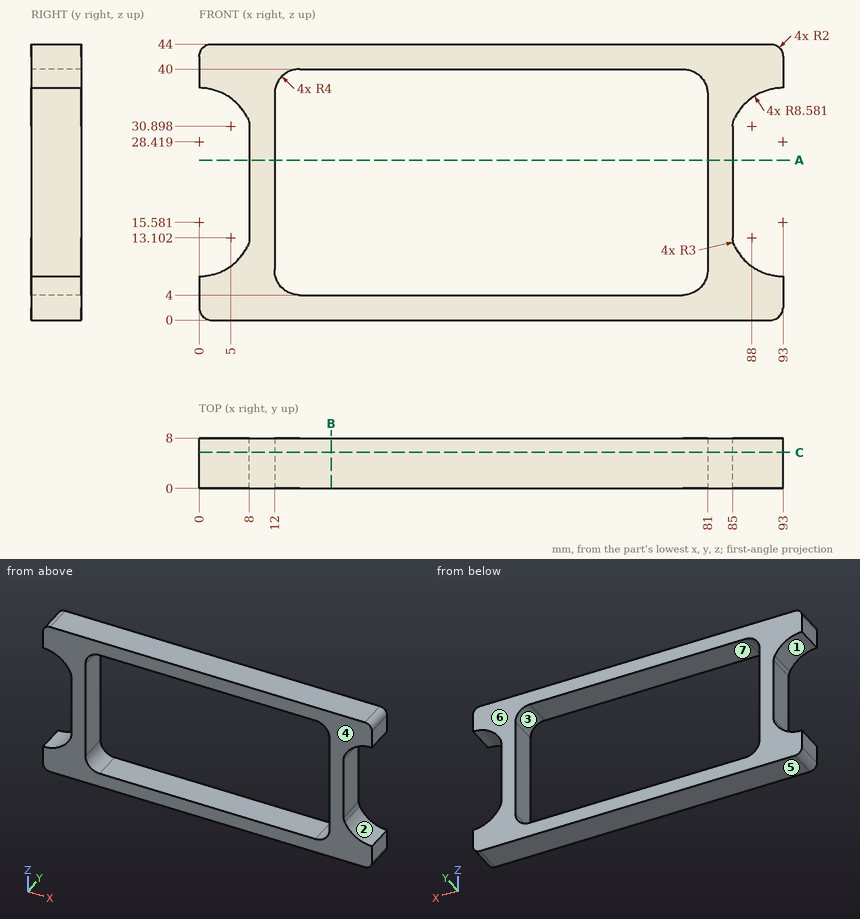
Could you check a few things on this drawing? It's one solid part, dimensions in mm from its lowest x, y, z. A direction names the side the tool comes from. Coordinates: 2 decimals unless noted, no trailing zeros. Order: outer loops, then holes, each group sorted by start corner. A loop starts at its lowest first (then second) coordinate and runs counter-clockwise, first axis right, second up. Notation, with made-up numbers: M 17.5,78 L 23.5,78 A12 ccw 23.5,88 Z; hole C 3,9.25 d2. An arc over 180 degrees is marked long. Answer as a JSON object with one key per item and string values. Group by question number.
(1) Which directions (+Z, -Z, +X, -X, +Y, -Y) give clear straight access to the entire face, cutting with the end or side of a thin tool? Please do the marked faces 1, 2, 3 and 4.
(2) For pin 1 (3 mm diameter, centred on y = 6, z = 23, fed in from -X); pin 2 (2.5 mm diameter, centred on y = 5.5, z = 21, fed in from +X), each with a flat end and sliding along its axis, tell me the tip position at first contact or that it passes through.
(3) I need wall thicknesses on probe 1 along Z at (x, y) = (31.5, 2.25); probe 2 along X at (y, z) = (2.5, 15.5); probe 3 along Z at (x, y) = (7, 3.75). Which ranges of each line are inside material? Lowest first, please.
(4) Suppose I cut it at A-A, the plane z = 25.5. Please give me the cut outline in (x, y).
(5) Suppose I cut it at B-B, the plane x = 21. Please give me the cut outline in (y, z).
(6) Suppose I cut it at C-C, the plane y = 5.75. Please give me the cut outline in (x, z), then the cut area to 3 significant figures.
(7) If we mould it in two halves opening along Z, with no side actions, what happens to the marked faces 5, 6 and 7? For each: released by +Z, released by -Z, zero draft, split by the parting line, or undercut.
Values found:
{
 "1": {"face 1": "-X, +Y, -Y", "face 2": "+X, +Y, -Y", "face 3": "+Y, -Y", "face 4": "+Z, -Z, +X, -X, -Y"},
 "2": {"pin 1": "stops at x = 8", "pin 2": "stops at x = 85"},
 "3": {"probe 1": "z = 0 to 4, 40 to 44", "probe 2": "x = 8 to 12, 81 to 85", "probe 3": "z = 0 to 10.62, 33.38 to 44"},
 "4": {"outline": "M 8,0 L 12,0 L 12,8 L 8,8 Z; M 81,0 L 85,0 L 85,8 L 81,8 Z"},
 "5": {"outline": "M 0,0 L 8,0 L 8,4 L 0,4 Z; M 0,40 L 8,40 L 8,44 L 0,44 Z"},
 "6": {"outline": "M 0,2 A2 ccw 2,0 L 91,0 A2 ccw 93,2 L 93,7 A8.58 cw 85.31,11.77 A3 cw 85,13.1 L 85,30.9 A3 cw 85.31,32.23 A8.58 cw 93,37 L 93,42 A2 ccw 91,44 L 2,44 A2 ccw 0,42 L 0,37 A8.58 cw 7.69,32.23 A3 cw 8,30.9 L 8,13.1 A3 cw 7.69,11.77 A8.58 cw 0,7 Z; hole M 12,8 A4 ccw 16,4 L 77,4 A4 ccw 81,8 L 81,36 A4 ccw 77,40 L 16,40 A4 ccw 12,36 Z", "area": "1,190 mm^2"},
 "7": {"face 5": "released by -Z", "face 6": "zero draft", "face 7": "undercut"}
}
